Read the model definition and answer for the solid it produces. Units are mm, in the model's axes. Give positions to 0.01 mm unless a question says otherwise; leave off trailing zeros. Order: outer loops, then holes, each group sorted by start corner. A loop starts at its lowest first (then second) coordinate and runs counter-clockwise, first axis right, second up. Notation, with made-up numbers: (23, -12.75) - (41, -12.75) arc R18 ccw to (41, 11.25) - close; hole circle Ø5 at (-8, 56). An arc over 180 degrees is marked (long way). Write item = value, one per line.
```python
from build123d import *

# Parameters (mm, degrees)
SKETCH1_W           = 51.9684
SKETCH1_H           = 48.0822
BOSS_EXTRUDE1_DEPTH = 7.8232
FILLET1_R           = 2.54
FILLET2_R           = 2.54
SKETCH3_R           = 1.5748
CUT_EXTRUDE1_DEPTH  = 72.230716785


with BuildPart() as part:
    # Sketch1 → Boss-Extrude1 (new body)
    with BuildSketch(Plane(origin=(0, 0, 0), x_dir=(1, 0, 0), z_dir=(0, 1, 0))):
        with Locations((25.9842, 24.0411)):
            Rectangle(SKETCH1_W, SKETCH1_H)
    extrude(amount=BOSS_EXTRUDE1_DEPTH)

    # Fillet1
    fillet1_edges = [part.edges().sort_by_distance(p)[0] for p in [
        (0, 3.9116, -48.0822),
        (51.9684, 3.9116, -48.0822),
        (51.9684, 3.9116, 0),
        (0, 3.9116, 0),
    ]]
    fillet(fillet1_edges, radius=FILLET1_R)

    # Fillet2
    # the kernel refuses this fillet: 2.54 mm, written as the material it takes off along each edge
    with BuildSketch(Plane(origin=(55.7784, 7.8232, -48.0822), x_dir=(0, 0, 1), z_dir=(-1, 0, 0))) as fillet2_piece_1:
        with BuildLine():
            CenterArc((FILLET2_R, -FILLET2_R), FILLET2_R, 90, 90)
            Line((0, -FILLET2_R), (0, 0))
            Line((0, 0), (FILLET2_R, 0))
        make_face()
    extrude(amount=59.5884, mode=Mode.SUBTRACT)

    # Sketch3 → Cut-Extrude1 (cut, through all)
    with BuildSketch(Plane(origin=(0, 7.8232, 0), x_dir=(1, 0, 0), z_dir=(0, 1, 0))):
        with Locations(Location((25.9842, 38.354, 0), (0, 0, 270))):
            Circle(SKETCH3_R)
    extrude(amount=-CUT_EXTRUDE1_DEPTH, mode=Mode.SUBTRACT)


solid = part.part
```
1. Section A-A (y = 7.25) is taken. Determine the outline of the cut face in (x, z).
Recorded:
outline = (0, -45.54) arc R2.54 ccw to (0.57, -47.15) - (51.4, -47.15) arc R2.54 ccw to (51.97, -45.54) - (51.97, -2.54) arc R2.54 ccw to (49.43, 0) - (2.54, 0) arc R2.54 ccw to (0, -2.54) - close; hole circle Ø3.15 at (25.98, -38.35)
2. Straight lines are drawn through the part: L1, parallel to X at y = 1.25, z = -38.5; L2, parallel to Z at x = 49.5, y = 5.5; L3, parallel to Z at x = 25, y = 5.5. For each, find the intervals that lie inside material, in ascending order. Write a range as [from, to].
Recorded:
L1 = [0, 24.42], [27.55, 51.97]
L2 = [-48.07, 0]
L3 = [-48.07, -39.58], [-37.12, 0]
3. Determine the mould class of faces 1 (the face through (0.724, 3.966, -0.764)), 2 (the face through (25.38, 3.97, -36.9)), 3 (the face through (51.2, 3.97, -0.72)) for opening direction X: +X half, -X half, draft (parallel to the pull), parting line (faces both ways), or undercut.
Recorded:
face_1 = -X half
face_2 = undercut
face_3 = +X half
